Can you work these out from the model? Positions are in its coordinate system, mm. A direction names the side the tool comes from. Give positions to 0.01 mm unless a question says otherwise; leave off trailing zeros. Order: outer loops, then holes, each group sorted by start corner. A loop starts at its lowest first (then second) coordinate and runs counter-clockwise, first axis right, second up.
Item 1: Which directions (+Z, -Z, +X, -X, +Y, -Y) give clear straight access to the entire face, cutting with the end or side of a thin tool? Please do faces 5 (the flat face through (4, -9, 32.5)), 6 (the cylindrical face through (-8.7, -5.5, 19)), 7 (the flat face through (10, 0, 14)), 8 (the flat face through (0, -10, 15)), 9 (the flat face through (10, 0, 18.5)).
Item 2: If we mould it in two halves opening along X, with no side actions, what happens to faces 1 (the cylindrical face through (-10.49, 0.46, 16.02)), 2 (the flat face through (-3.4, -10.2, 0)), 3 (the cylindrical face through (-5.5, 8.7, 17)), 4 (the cylindrical face through (-9.24, 0.41, 15.74))? For each: +X half, -X half, draft (parallel to the pull), parting line (faces both ways), or undercut.
Item 3: I'm going to push flat-ended pins straight in: pin 1 Ø3 at (x, z) = (-5.5, 13) entering from +Y; pin 2 Ø3 at (y, z) = (-7.5, 18) entering from +X; pin 3 Ø4 at (y, z) = (-2.5, 10) entering from -X; pin 4 Ø4 at (x, y) = (7, -4) entering from +Z. Where does each tip first touch, or does it pass through?
Item 4: I want a section at A-A, the plane x = 0. Write out the boundary of the cut face in (y, z), then the cut area to 3 significant figures.
Item 5: I want a section at C-C, the plane x = 5.25. Write out the boundary of the cut face in (y, z).
Item 6: If I drill on line 1 along Y through (x, z) = (0, 14.5); line 2 along Z through (x, y) = (-9.5, -3.5); line 3 along Z through (x, y) = (9, -2.5), over which ranges is the centre line in solid material (lowest first)?
Item 7: I want a section at B-B, the plane y = 1.5. Write out the boundary of the cut face in (x, z).
Item 8: I want a section at D-D, the plane z = 27.5. Write out the boundary of the cut face in (x, y).
```python
from build123d import *

# Parameters (mm, degrees)
ESQUISSE1_R             = 10.5
BASE_EXTRUSION_DEPTH    = 32.5
ESQUISSE3_R             = 11.5
BOSS_EXTRU_1_DEPTH      = 1.5
ESQUISSE2_R             = 9.25
ENL_V_MAT_EXTRU_1_DEPTH = 38.68952109
ENL_V_MAT_EXTRU_2_REACH = 42.896
ENL_V_MAT_EXTRU_3_DEPTH = 41.896210173
ENL_V_MAT_EXTRU_5_REACH = 43.167


with BuildPart() as part:
    # Esquisse1 → Base-Extrusion (new body)
    with BuildSketch(Plane.XY):
        Circle(ESQUISSE1_R)
    extrude(amount=BASE_EXTRUSION_DEPTH)

    # Esquisse3 → Boss.-Extru.1 (add)
    with BuildSketch(Plane(origin=(0, 0, 0), x_dir=(-1, 0, 0), z_dir=(0, 0, -1))):
        Circle(ESQUISSE3_R)
    extrude(amount=BOSS_EXTRU_1_DEPTH)

    # Esquisse2 → Enlèv. mat.-Extru.1 (cut, through all)
    with BuildSketch(Plane.XY.offset(32.5)):
        Circle(ESQUISSE2_R)
    extrude(amount=-ENL_V_MAT_EXTRU_1_DEPTH, mode=Mode.SUBTRACT)

    # Esquisse4 → Enlèv. mat.-Extru.2 (cut, up to next)
    with BuildSketch(Plane(origin=(10.5, 0, 0), x_dir=(0, 0, -1), z_dir=(1, 0, 0)), mode=Mode.PRIVATE) as enl_v_mat_extru_2_sk1:
        with BuildLine():
            Line((-14, 4.75), (-14, -4.75))
            ThreePointArc((-14, -4.75), (-16.25, -7), (-18.5, -4.75))
            Line((-18.5, -4.75), (-18.5, 4.75))
            ThreePointArc((-18.5, 4.75), (-16.25, 7), (-14, 4.75))
        make_face()
    enl_v_mat_extru_2_tool1 = extrude(enl_v_mat_extru_2_sk1.sketch, amount=-ENL_V_MAT_EXTRU_2_REACH, mode=Mode.PRIVATE) & part.part
    add(enl_v_mat_extru_2_tool1.solids().sort_by_distance((10.5, 0, 16.25))[0], mode=Mode.SUBTRACT)

    # Esquisse5 → Enlèv. mat.-Extru.3 (cut, through all)
    with BuildSketch(Plane(origin=(0, 10.5, 0), x_dir=(-1, 0, 0), z_dir=(0, 1, 0))):
        with BuildLine():
            Line((3.5, 19), (-2.5, 19))
            ThreePointArc((-2.5, 19), (-4.5, 17), (-2.5, 15))
            Line((-2.5, 15), (3.5, 15))
            ThreePointArc((3.5, 15), (5.5, 17), (3.5, 19))
        make_face()
    extrude(amount=-ENL_V_MAT_EXTRU_3_DEPTH, mode=Mode.SUBTRACT)

    # Esquisse7 → Enlèv. mat.-Extru.5 (cut, up to next)
    with BuildSketch(Plane(origin=(-11, 0, 0), x_dir=(0, 0, -1), z_dir=(1, 0, 0)), mode=Mode.PRIVATE) as enl_v_mat_extru_5_sk1:
        with BuildLine():
            Line((-17, -3.5), (-17, 3.5))
            ThreePointArc((-17, 3.5), (-19, 5.5), (-21, 3.5))
            Line((-21, 3.5), (-21, -3.5))
            ThreePointArc((-21, -3.5), (-19, -5.5), (-17, -3.5))
        make_face()
    enl_v_mat_extru_5_tool1 = extrude(enl_v_mat_extru_5_sk1.sketch, amount=ENL_V_MAT_EXTRU_5_REACH, mode=Mode.PRIVATE) & part.part
    add(enl_v_mat_extru_5_tool1.solids().sort_by_distance((-11, 0, 19))[0], mode=Mode.SUBTRACT)


solid = part.part
```
Results list:
1. face 5: +Z, +X, -X, +Y, -Y
1. face 6: -X
1. face 7: +X
1. face 8: +Y, -Y
1. face 9: +X, -X
2. face 1: parting line
2. face 2: draft
2. face 3: undercut
2. face 4: undercut
3. pin 1: stops at y = 9.71
3. pin 2: stops at x = 8.61
3. pin 3: stops at x = -10.49
3. pin 4: stops at z = 32.5
4. outline: (-11.5, -1.5) - (-9.25, -1.5) - (-9.25, 15) - (-10.5, 15) - (-10.5, 0) - (-11.5, 0) - close; (-10.5, 19) - (-9.25, 19) - (-9.25, 32.5) - (-10.5, 32.5) - close; (9.25, -1.5) - (11.5, -1.5) - (11.5, 0) - (10.5, 0) - (10.5, 15) - (9.25, 15) - close; (9.25, 19) - (10.5, 19) - (10.5, 32.5) - (9.25, 32.5) - close
4. area: 78.0 mm2
5. outline: (-10.23, -1.5) - (-7.62, -1.5) - (-7.62, 32.5) - (-9.09, 32.5) - (-9.09, 0) - (-10.23, 0) - close; (7.62, -1.5) - (10.23, -1.5) - (10.23, 0) - (9.09, 0) - (9.09, 32.5) - (7.62, 32.5) - close
6. line 1: y = -10.5 to -9.25, 9.25 to 10.5
6. line 2: z = -1.5 to 17, 21 to 32.5
6. line 3: z = -1.5 to 14, 18.5 to 32.5
7. outline: (-11.4, -1.5) - (-9.13, -1.5) - (-9.13, 17) - (-10.39, 17) - (-10.39, 0) - (-11.4, 0) - close; (-10.39, 21) - (-9.13, 21) - (-9.13, 32.5) - (-10.39, 32.5) - close; (9.13, -1.5) - (11.4, -1.5) - (11.4, 0) - (10.39, 0) - (10.39, 14) - (9.13, 14) - close; (9.13, 18.5) - (10.39, 18.5) - (10.39, 32.5) - (9.13, 32.5) - close
8. outline: circle Ø21 at (0, 0); hole circle Ø18.5 at (0, 0)
